```python
from build123d import *

# Parameters (mm, degrees)
SKETCH_R     = 3.2
PAD_DEPTH    = 3
SKETCH001_W  = 2.54
SKETCH001_H  = 38.1
PAD001_DEPTH = 44
SKETCH002_R  = 3.2
PAD002_DEPTH = 3
FILLET_R     = 3


with BuildPart() as part:
    # Sketch → Pad (new body)
    with BuildSketch(Plane.XY):
        with BuildLine():
            Line((-12.7, 19.05), (12.7, 19.05))
            ThreePointArc((19.05, 12.7), (17.190128, 17.190128), (12.7, 19.05))
            Line((19.05, 12.7), (19.05, -12.7))
            ThreePointArc((12.7, -19.05), (17.190128, -17.190128), (19.05, -12.7))
            Line((12.7, -19.05), (-12.7, -19.05))
            ThreePointArc((-19.05, -12.7), (-17.190128, -17.190128), (-12.7, -19.05))
            Line((-19.05, -12.7), (-19.05, 12.7))
            ThreePointArc((-12.7, 19.05), (-17.190128, 17.190128), (-19.05, 12.7))
        make_face()
        with Locations((-12.7, 12.7)):
            Circle(SKETCH_R, mode=Mode.SUBTRACT)
        with Locations((12.7, 12.7)):
            Circle(SKETCH_R, mode=Mode.SUBTRACT)
        with Locations((12.7, -12.7)):
            Circle(SKETCH_R, mode=Mode.SUBTRACT)
        with Locations((-12.7, -12.7)):
            Circle(SKETCH_R, mode=Mode.SUBTRACT)
    extrude(amount=PAD_DEPTH)

    # Sketch001 (on Face14 of Pad) → Pad001 (join)
    with BuildSketch(Plane.XY.offset(3)):
        with Locations((-5.83, 0)):
            Rectangle(SKETCH001_W, SKETCH001_H)
        with Locations((5.83, 0)):
            Rectangle(SKETCH001_W, SKETCH001_H)
    extrude(amount=PAD001_DEPTH)

    # Sketch002 (on Face22 of Pad001) → Pad002 (join)
    with BuildSketch(Plane.XY.offset(47)):
        with BuildLine():
            Line((-12.7, 19.05), (12.7, 19.05))
            ThreePointArc((19.05, 12.7), (17.190128, 17.190128), (12.7, 19.05))
            Line((19.05, 12.7), (19.05, -12.7))
            ThreePointArc((12.7, -19.05), (17.190128, -17.190128), (19.05, -12.7))
            Line((12.7, -19.05), (-12.7, -19.05))
            ThreePointArc((-19.05, -12.7), (-17.190128, -17.190128), (-12.7, -19.05))
            Line((-19.05, -12.7), (-19.05, 12.7))
            ThreePointArc((-12.7, 19.05), (-17.190128, 17.190128), (-19.05, 12.7))
        make_face()
        with Locations((-12.7, 12.7)):
            Circle(SKETCH002_R, mode=Mode.SUBTRACT)
        with Locations((12.7, 12.7)):
            Circle(SKETCH002_R, mode=Mode.SUBTRACT)
        with Locations((12.7, -12.7)):
            Circle(SKETCH002_R, mode=Mode.SUBTRACT)
        with Locations((-12.7, -12.7)):
            Circle(SKETCH002_R, mode=Mode.SUBTRACT)
    extrude(amount=PAD002_DEPTH)

    # Fillet
    fillet_edges = [part.edges().sort_by_distance(p)[0] for p in [
        (4.56, 0, 3),
        (-7.1, 0, 3),
        (-4.56, 0, 3),
        (7.1, 0, 3),
        (7.1, 0, 47),
        (-4.56, 0, 47),
        (4.56, 0, 47),
        (-7.1, 0, 47),
    ]]
    fillet(fillet_edges, radius=FILLET_R)


solid = part.part
```
Build history of the part. All positions in model axes, mm. A direction names the side the tool comes from. Give positions to 0.01 mm unless a question says otherwise; leave off trailing zeros. Loops run counter-clockwise (first coordinate to the right, second up) from the corner with the lowest first, then second, coordinate; pieces in that order, holes last.
1) Band-saw the part on B-B on y = -4.5. List the corners of the cut face in (x, z).
Values follow:
outline: (-19.05, 0) - (19.05, 0) - (19.05, 3) - (10.1, 3) arc R3 cw to (7.1, 6) - (7.1, 44) arc R3 cw to (10.1, 47) - (19.05, 47) - (19.05, 50) - (-19.05, 50) - (-19.05, 47) - (-10.1, 47) arc R3 cw to (-7.1, 44) - (-7.1, 6) arc R3 cw to (-10.1, 3) - (-19.05, 3) - close; hole (-4.56, 6) arc R3 ccw to (-1.56, 3) - (1.56, 3) arc R3 ccw to (4.56, 6) - (4.56, 44) arc R3 ccw to (1.56, 47) - (-1.56, 47) arc R3 ccw to (-4.56, 44) - close
2) Probe line 1 along Y through (x, z) = (12.7, 48.15); line 2 along X through (y, z) = (13, 2); line 3 along Z through (x, y) = (0.5, 2.5). List the from-to ranges inside material, lowest first.
Values follow:
line 1: y = -19.05 to -15.9, -9.5 to 9.5, 15.9 to 19.05
line 2: x = -19.04 to -15.89, -9.51 to 9.51, 15.89 to 19.04
line 3: z = 0 to 3, 47 to 50
3) 3-axis set-ups, long thin cutter, end or side, ignore diameter. For faces 4 (the face through (7.96, -16.78, 3.9)), 5 (the face through (0, 0, 47)), 6 (the face through (-7.96, -16.78, 3.9)), 7 (the face through (-15.06, 14.86, 1.48)): which of +Z, -Z, +X, -X, +Y, -Y reach the whole face in a straight line?
Values follow:
face 4: +X, +Y, -Y
face 5: +Y, -Y
face 6: -X, +Y, -Y
face 7: +Z, -Z
4) Band-saw the part on A-A on z = 21.5. List the corners of the cut face in (x, y), then the cut area to 3 significant figures.
Values follow:
outline: (-7.1, -19.05) - (-4.56, -19.05) - (-4.56, 19.05) - (-7.1, 19.05) - close; (4.56, -19.05) - (7.1, -19.05) - (7.1, 19.05) - (4.56, 19.05) - close
area: 194 mm2
5) Drop flat-ended pins along their axis: P1, Ø1.5, axis at x = 11.5, y = 10, coming from the +Z side; P2, Ø5, axis at y = -5.5, z = 43.5, coming from the +X side; P3, Ø5, axis at x = -12.7, y = 12.7, coming from the -Z side. Give the stop position or say it passes through.
Values follow:
P1: stops at z = 50
P2: stops at x = 7.86
P3: passes through
6) Band-saw the part on C-C on x = 2.5. List the corners of the cut face in (y, z).
Values follow:
outline: (-19.05, 0) - (19.05, 0) - (19.05, 3.15) - (-19.05, 3.15) - close; (-19.05, 46.85) - (19.05, 46.85) - (19.05, 50) - (-19.05, 50) - close
7) Two-plate mould, pull along Z, no slides. Class faces 1 (the face through (4.56, 0, 25)), 2 (the face through (0, 0, 0)), 3 (the face through (17.24, 17.14, 48.48)): released by +Z, released by -Z, zero draft, split by the parting line, or undercut.
Values follow:
face 1: undercut
face 2: released by -Z
face 3: zero draft
